Build history of the part. All positions in model axes, mm. A direction names the side the tool comes from. Round coordinates to 2 decimals unless told otherwise and drop trailing zeros. Order: outer loops, then holes, each group sorted by start corner. A loop starts at its lowest first (then second) coordinate and runs counter-clockwise, first axis right, second up. Notation, with made-up numbers: (52.5, 15) -> (100.5, 15) arc R20 ccw to (100.5, 50) -> close; hole circle Ø10 at (18, 25). An arc over 180 degrees is marked (long way). Use a Markdown table: item, result. Add a question column.
Item 1: Slice it at D-D, the plane y = -32.7. Give the cut face in (x, z).
Item 2: Slice it at A-A, the plane y = -21.5. Give the cut face in (x, z), plus the area to 3 significant figures.
Item 3: 3-axis set-ups, long thin cutter, end or side, ignore diameter. For faces 5 (the face through (-13, -3, 5)), 6 (the face through (10.195, -34.187, 9.274)), 7 (the face through (-13, -42, 5)), 8 (the face through (0, -22, 5)): which of +Z, -Z, +X, -X, +Y, -Y reach the whole face in a straight line?
Item 4: Slice it at C-C, the plane z = 9.75. Give the cut face in (x, y), plus the area to 3 significant figures.
Item 5: Two-plate mould, pull along Y, no slides. Class faces 1 (the face through (0, -45.4, 6)), 2 (the face through (-9, -22, 11)), 3 (the face through (0, 0, 6)), 4 (the face through (-9.805, -34.187, 9.274)): released by +Y, released by -Y, zero draft, split by the parting line, or undercut.
Item 6: Pin check, flat tips, straight feed: pin 1 (0.9 mm diameter, centred on x = 10.5, y = -32, fed in from +Z); pin 2 (3 mm diameter, centred on y = -42.5, z = 5, fed in from +X); pin 3 (3.5 mm diameter, centred on x = 1, y = -29.5, fed in from -Z). Stop position of each tip, or through.
Item 7: Slice it at B-B, the plane x = 10. Give the cut face in (y, z), plus the area to 3 significant figures.
Item 8: Probe L1, parallel to X at y = -12.7, z = 9.2; L2, parallel to Y at x = 10, z = 8.7; L3, parallel to Y at x = 9.5, z = 8. List the from-to ranges inside material, lowest first.
from build123d import *

# Parameters (mm, degrees)
PAD_DEPTH       = 45.4
SKETCH001_R     = 1.5
POCKET_DEPTH    = 3.5
SKETCH002_W     = 27
SKETCH002_H     = 6.5
POCKET001_DEPTH = 0.5
SKETCH003_W     = 10.5
SKETCH003_H     = 6.5
POCKET002_DEPTH = 0.5
SKETCH004_W     = 10
SKETCH004_H     = 32.4
POCKET003_DEPTH = 0.5


with BuildPart() as part:
    # Sketch → Pad (new body)
    with BuildSketch(Plane.XZ):
        with BuildLine():
            Line((-13, 0), (-6, 0))
            Line((-6, 0), (-6, 5))
            Line((-6, 5), (6, 5))
            Line((6, 5), (6, 0))
            Line((6, 0), (13, 0))
            ThreePointArc((13, 0), (13.353553, 0.146447), (13.5, 0.5))
            Line((13.5, 0.5), (13.5, 10.5))
            ThreePointArc((13.5, 10.5), (13.353553, 10.853553), (13, 11))
            Line((-13, 11), (13, 11))
            ThreePointArc((-13, 11), (-13.353553, 10.853553), (-13.5, 10.5))
            Line((-13.5, 0.5), (-13.5, 10.5))
            ThreePointArc((-13.5, 0.5), (-13.353553, 0.146447), (-13, 0))
        make_face()
    extrude(amount=PAD_DEPTH)

    # Sketch001 (on Face10 of Pad) → Pocket (cut)
    with BuildSketch(Plane(origin=(0, 0, 11), x_dir=(-1, 0, 0), z_dir=(0, 0, 1))):
        with Locations((-10, 12.7)):
            Circle(SKETCH001_R)
        with Locations((10, 12.7)):
            Circle(SKETCH001_R)
        with Locations((-10, 32.7)):
            Circle(SKETCH001_R)
        with Locations((10, 32.7)):
            Circle(SKETCH001_R)
    extrude(amount=-POCKET_DEPTH, mode=Mode.SUBTRACT)

    # Sketch002 (on Face14 of Pocket) → Pocket001 (cut)
    with BuildSketch(Plane(origin=(0, 0, 11), x_dir=(-1, 0, 0), z_dir=(0, 0, 1))):
        with Locations((0, 3.25)):
            Rectangle(SKETCH002_W, SKETCH002_H)
        with Locations((0, 42.15)):
            Rectangle(SKETCH002_W, SKETCH002_H)
    extrude(amount=-POCKET001_DEPTH, mode=Mode.SUBTRACT)

    # Sketch003 (on Face10 of Pocket001) → Pocket002 (cut)
    with BuildSketch(Plane(origin=(13.5, 0, 0), x_dir=(0, 0, 1), z_dir=(1, 0, 0))):
        with Locations((5.25, 42.15)):
            Rectangle(SKETCH003_W, SKETCH003_H)
        with Locations((5.25, 3.25)):
            Rectangle(SKETCH003_W, SKETCH003_H)
    pocket002 = extrude(amount=-POCKET002_DEPTH, mode=Mode.SUBTRACT)

    # Mirrored: Pocket002 across YZ
    add(pocket002.mirror(Plane.YZ), mode=Mode.SUBTRACT)

    # Sketch004 (on Face24 of Mirrored) → Pocket003 (cut)
    with BuildSketch(Plane(origin=(0, 0, 11), x_dir=(-1, 0, 0), z_dir=(0, 0, 1))):
        with Locations((0, 22.7)):
            Rectangle(SKETCH004_W, SKETCH004_H)
    extrude(amount=-POCKET003_DEPTH, mode=Mode.SUBTRACT)


solid = part.part
Check sheet entries:
| question | item | result |
|---|---|---|
| 1 | outline | (-13.5, 0.5) arc R0.5 ccw to (-13, 0) -> (-6, 0) -> (-6, 5) -> (6, 5) -> (6, 0) -> (13, 0) arc R0.5 ccw to (13.5, 0.5) -> (13.5, 10.5) arc R0.5 ccw to (13, 11) -> (11.5, 11) -> (11.5, 7.5) -> (8.5, 7.5) -> (8.5, 11) -> (5, 11) -> (5, 10.5) -> (-5, 10.5) -> (-5, 11) -> (-8.5, 11) -> (-8.5, 7.5) -> (-11.5, 7.5) -> (-11.5, 11) -> (-13, 11) arc R0.5 ccw to (-13.5, 10.5) -> close |
| 2 | outline | (-13.5, 0.5) arc R0.5 ccw to (-13, 0) -> (-6, 0) -> (-6, 5) -> (6, 5) -> (6, 0) -> (13, 0) arc R0.5 ccw to (13.5, 0.5) -> (13.5, 10.5) arc R0.5 ccw to (13, 11) -> (5, 11) -> (5, 10.5) -> (-5, 10.5) -> (-5, 11) -> (-13, 11) arc R0.5 ccw to (-13.5, 10.5) -> close |
| 2 | area | 232 mm2 |
| 3 | face 5 | +Z, -Z, -X, +Y |
| 3 | face 6 | +Z |
| 3 | face 7 | +Z, -Z, -X, -Y |
| 3 | face 8 | -Z, +Y, -Y |
| 4 | outline | (-13.5, -38.9) -> (-13, -38.9) -> (-13, -45.4) -> (13, -45.4) -> (13, -38.9) -> (13.5, -38.9) -> (13.5, -6.5) -> (13, -6.5) -> (13, 0) -> (-13, 0) -> (-13, -6.5) -> (-13.5, -6.5) -> close; hole circle Ø3 at (-10, -32.7); hole circle Ø3 at (-10, -12.7); hole circle Ø3 at (10, -32.7); hole circle Ø3 at (10, -12.7) |
| 4 | area | 1,180 mm2 |
| 5 | face 1 | released by -Y |
| 5 | face 2 | zero draft |
| 5 | face 3 | released by +Y |
| 5 | face 4 | undercut |
| 6 | pin 1 | z = 7.5 |
| 6 | pin 2 | x = 13 |
| 6 | pin 3 | z = 5 |
| 7 | outline | (-45.4, 0) -> (0, 0) -> (0, 10.5) -> (-6.5, 10.5) -> (-6.5, 11) -> (-11.2, 11) -> (-11.2, 7.5) -> (-14.2, 7.5) -> (-14.2, 11) -> (-31.2, 11) -> (-31.2, 7.5) -> (-34.2, 7.5) -> (-34.2, 11) -> (-38.9, 11) -> (-38.9, 10.5) -> (-45.4, 10.5) -> close |
| 7 | area | 472 mm2 |
| 8 | L1 | -13.5 to -11.5, -8.5 to 8.5, 11.5 to 13.5 |
| 8 | L2 | -45.4 to -34.2, -31.2 to -14.2, -11.2 to 0 |
| 8 | L3 | -45.4 to -34.11, -31.29 to -14.11, -11.29 to 0 |
